Work out the finished part from the listing and answer in its coordinate system (mm). Give positions to 0.01 mm unless a question says otherwise; leave off trailing zeros. Loops run counter-clockwise (first coordinate to the right, second up) from the corner with the lowest first, then second, coordinate; pieces in that order, holes last. Notation, with made-up numbers: M -31,73 L -21,73 A23 ccw -21,95 Z; hole C 3.5,66 d4. An arc over 180 degrees is marked long. Use a Markdown table: item, result.
```python
from build123d import *

# Parameters (mm, degrees)
SKETCH1_R             = 16.5
EXTRUDE1_DEPTH        = 1.016
F_0_CLEARANCE_HOLE1_D = 1.6129
SKETCH6_R             = 0.80645
CUT_EXTRUDE1_DEPTH    = 5


with BuildPart() as part:
    # Sketch1 → Extrude1 (new body)
    with BuildSketch(Plane.XY):
        Circle(SKETCH1_R)
    extrude(amount=EXTRUDE1_DEPTH)

    # #0 Clearance Hole1 (through all)
    with Locations(Plane(origin=(0, 10, 0), x_dir=(-1, 0, 0), z_dir=(0, 0, -1))):
        with Locations((0, 0), (8.660254038, -15), (-8.660254038, -15)):
            Hole(F_0_CLEARANCE_HOLE1_D / 2)

    # Sketch6 → Cut-Extrude1 (cut)
    with BuildSketch(Plane.XY.offset(1.016)):
        with Locations((0, 15)):
            Circle(SKETCH6_R)
        with Locations((12.990381057, -7.5)):
            Circle(SKETCH6_R)
        with Locations((-12.990381057, -7.5)):
            Circle(SKETCH6_R)
    extrude(amount=-CUT_EXTRUDE1_DEPTH, mode=Mode.SUBTRACT)


solid = part.part
```
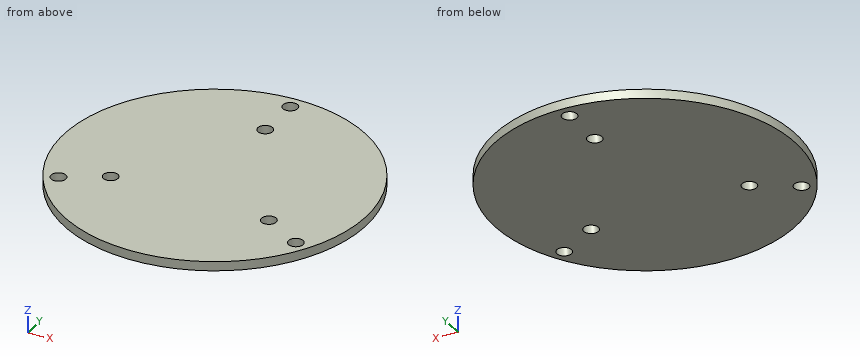
(1) A cutting plane is placed at D-D (y = 15). Write down the section's boundary in (x, z).
Entries:
| item | result |
|---|---|
| outline | M -6.87,0 L -0.81,0 L -0.81,1.02 L -6.87,1.02 Z; M 0.81,0 L 6.87,0 L 6.87,1.02 L 0.81,1.02 Z |
(2) A cutting plane is placed at C-C (y = -5). Write down the section's boundary in (x, z).
Entries:
| item | result |
|---|---|
| outline | M -15.72,0 L -9.47,0 L -9.47,1.02 L -15.72,1.02 Z; M -7.85,0 L 7.85,0 L 7.85,1.02 L -7.85,1.02 Z; M 9.47,0 L 15.72,0 L 15.72,1.02 L 9.47,1.02 Z |
(3) A cutting plane is placed at B-B (y = 10). Write down the section's boundary in (x, z).
Entries:
| item | result |
|---|---|
| outline | M -13.12,0 L -0.81,0 L -0.81,1.02 L -13.12,1.02 Z; M 0.81,0 L 13.12,0 L 13.12,1.02 L 0.81,1.02 Z |
(4) Consider probe 1 along Y at (x, z) = (0, 0.35); probe 2 along Y at (x, z) = (-13.5, 0.8); probe 3 along X at (y, z) = (14.5, 0.6). Determine where each line is inside the solid, lowest interval first. Write a range as [from, to].
Entries:
| item | result |
|---|---|
| probe 1 | y = [-16.5, 9.19], [10.81, 14.19], [15.81, 16.5] |
| probe 2 | y = [-9.49, -8.13], [-6.87, 9.49] |
| probe 3 | x = [-7.87, -0.63], [0.63, 7.87] |
(5) Given P1, Ø1.3, axis at x = 8.66, y = -5, coming from the -Z side, flat-ended and moving along its own axis, determine where the tip first touches the part or whether it passes through.
Entries:
| item | result |
|---|---|
| P1 | passes through |
(6) A cutting plane is placed at A-A (z = 0.4). Write down the section's boundary in (x, y), and give its area (3 significant figures).
Entries:
| item | result |
|---|---|
| outline | C 0,0 d33; hole C -12.99,-7.5 d1.61; hole C -8.66,-5 d1.61; hole C 0,10 d1.61; hole C 0,15 d1.61; hole C 8.66,-5 d1.61; hole C 12.99,-7.5 d1.61 |
| area | 843 mm² |
